Design review of the part shown in the three views and the two pictorial views. Dimensions are in mm from the part's minimum x, y and z. Round coordinates to 2 decimals unless told otherwise and drop trailing zeros. Order: outer loops, then holes, each group sorted by start corner. A loop starts at its lowest first (then second) coordinate and runs counter-clockwise, first axis right, second up. Notation, with made-up numbers: M 56.5,2.25 L 107.5,2.25 A14 cw 107.5,16.25 Z; hole C 23.5,83 d4. An arc over 180 degrees is marked long. Write item = value, one per line. Start each with the question number.
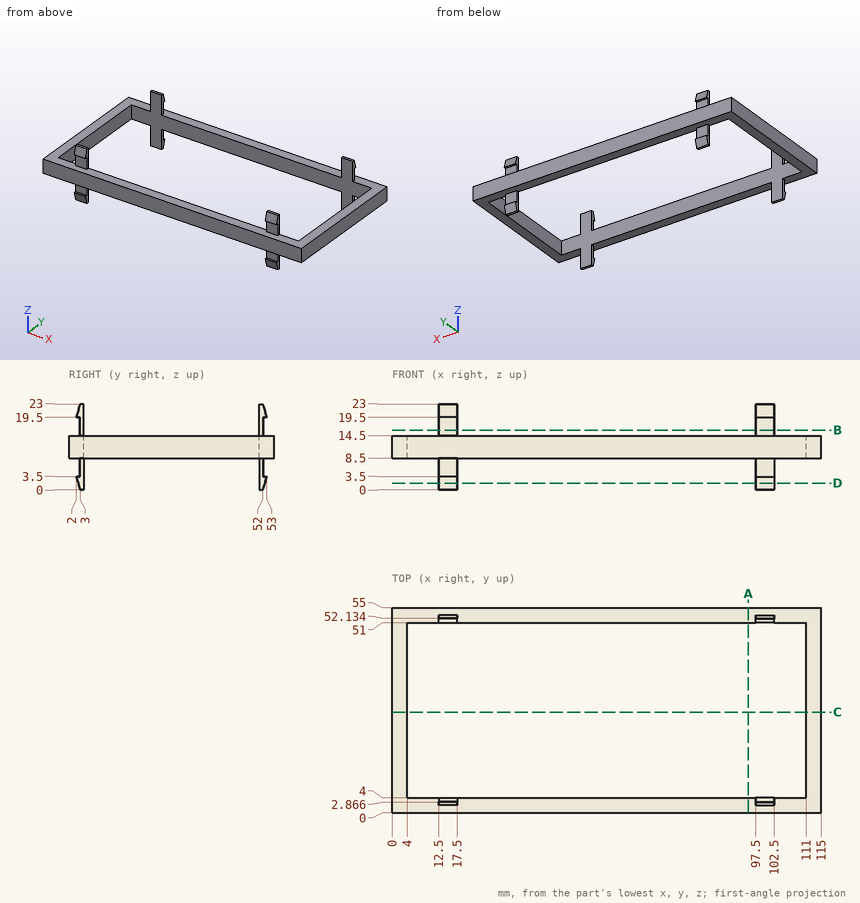
(1) We need section A-A, the plane x = 95.5. Write out the cut boundary in (y, z), then the cut area to 3 significant figures.
(2) We need section C-C, the plane y = 27. Write out the cut boundary in (x, z).
(3) We need section D-D, the plane z = 1.75. Write out the cut boundary in (x, y), then the cut area to 3 significant figures.
(4) We need section B-B, the plane z = 16. Write out the cut boundary in (x, y), then the cut area to 3 significant figures.
(5) Insertion check: pin 1 (2 mm diameter, centred on y = 3, z = 3, fed in from +X); pin 2 (1 mm diameter, centred on x = 24, z = 16.5, fed in from +Y); pin 3 (1.5 mm diameter, centred on y = 49.5, z = 14.5, fed in from -X); pin 4 (1 mm diameter, centred on y = 51.5, z = 17.5, fed in from -X). Each pin has a flat end and moves straight along its axis. Give the tip position at first contact, or say it passes through.
(6) For line 1 along Y through (x, z) = (44, 14), list the stretches that pass through material, from the lowest coordinate up.
Values:
q1.outline = M 0,8.5 L 4,8.5 L 4,14.5 L 0,14.5 Z; M 51,8.5 L 55,8.5 L 55,14.5 L 51,14.5 Z
q1.area = 48.0 mm²
q2.outline = M 0,8.5 L 4,8.5 L 4,14.5 L 0,14.5 Z; M 111,8.5 L 115,8.5 L 115,14.5 L 111,14.5 Z
q3.outline = M 12.5,2.5 L 17.5,2.5 L 17.5,4 L 12.5,4 Z; M 12.5,51 L 17.5,51 L 17.5,52.5 L 12.5,52.5 Z; M 97.5,2.5 L 102.5,2.5 L 102.5,4 L 97.5,4 Z; M 97.5,51 L 102.5,51 L 102.5,52.5 L 97.5,52.5 Z
q3.area = 30.0 mm²
q4.outline = M 12.5,2.87 L 17.5,2.87 L 17.5,4 L 12.5,4 Z; M 12.5,51 L 17.5,51 L 17.5,52.13 L 12.5,52.13 Z; M 97.5,2.87 L 102.5,2.87 L 102.5,4 L 97.5,4 Z; M 97.5,51 L 102.5,51 L 102.5,52.13 L 97.5,52.13 Z
q4.area = 22.7 mm²
q5.pin_1 = 102.5
q5.pin_2 = through
q5.pin_3 = 0
q5.pin_4 = 12.5
q6.line_1 = 0 to 4, 51 to 55
